```python
from build123d import *

# Parameters (mm, degrees)
SKETCH1_W           = 46
SKETCH1_H           = 21
BOSS_EXTRUDE1_DEPTH = 1
SKETCH2_W           = 21
SKETCH2_H           = 12
SKETCH2_W_2         = 11
SKETCH2_H_2         = 6
BOSS_EXTRUDE2_DEPTH = 4.5
SKETCH3_W           = 7.849871035
SKETCH3_H           = 3.412332869
CUT_EXTRUDE1_DEPTH  = 4
SKETCH4_R           = 5.109251927
BOSS_EXTRUDE3_DEPTH = 3
SKETCH5_R           = 1.986847175
CUT_EXTRUDE2_DEPTH  = 1.5
FILLET1_R           = 1
SKETCH6_R           = 1.1
CUT_EXTRUDE3_DEPTH  = 1.5


with BuildPart() as part:
    # Sketch1 → Boss-Extrude1 (new body)
    with BuildSketch(Plane(origin=(0, 0, 0), x_dir=(1, 0, 0), z_dir=(0, 1, 0))):
        with Locations((23, -10.5)):
            Rectangle(SKETCH1_W, SKETCH1_H)
    extrude(amount=BOSS_EXTRUDE1_DEPTH)

    # Sketch2 → Boss-Extrude2 (add)
    with BuildSketch(Plane(origin=(0, 1, 0), x_dir=(1, 0, 0), z_dir=(0, 1, 0))):
        with Locations((23, -10.5)):
            Rectangle(SKETCH2_W, SKETCH2_H)
        with Locations((39.939580859, -17.520481264)):
            Rectangle(SKETCH2_W_2, SKETCH2_H_2)
    extrude(amount=BOSS_EXTRUDE2_DEPTH)

    # Sketch3 → Cut-Extrude1 (cut)
    with BuildSketch(Plane.XY.offset(20.520481264)):
        with Locations((40.122531197, 3.793833565)):
            Rectangle(SKETCH3_W, SKETCH3_H)
    extrude(amount=-CUT_EXTRUDE1_DEPTH, mode=Mode.SUBTRACT)

    # Sketch4 → Boss-Extrude3 (add)
    with BuildSketch(Plane(origin=(0, 5.5, 0), x_dir=(1, 0, 0), z_dir=(0, 1, 0))):
        with Locations((23.147185082, -10.671715929)):
            Circle(SKETCH4_R)
    extrude(amount=BOSS_EXTRUDE3_DEPTH)

    # Sketch5 → Cut-Extrude2 (cut)
    with BuildSketch(Plane(origin=(0, 8.5, 0), x_dir=(1, 0, 0), z_dir=(0, 1, 0))):
        with Locations((23.147185082, -10.671715929)):
            Circle(SKETCH5_R)
    extrude(amount=-CUT_EXTRUDE2_DEPTH, mode=Mode.SUBTRACT)

    # Fillet1
    fillet1_edges = [part.edges().sort_by_distance(p)[0] for p in [
        (21.160337907, 8.5, 10.671715929),
    ]]
    fillet(fillet1_edges, radius=FILLET1_R)

    # Sketch6 → Cut-Extrude3 (cut)
    with BuildSketch(Plane(origin=(0, 1, 0), x_dir=(1, 0, 0), z_dir=(0, 1, 0))):
        with Locations((1.658163122, -10.5)):
            Circle(SKETCH6_R)
        with Locations((44.341836878, -10.5)):
            Circle(SKETCH6_R)
    extrude(amount=-CUT_EXTRUDE3_DEPTH, mode=Mode.SUBTRACT)


solid = part.part
```
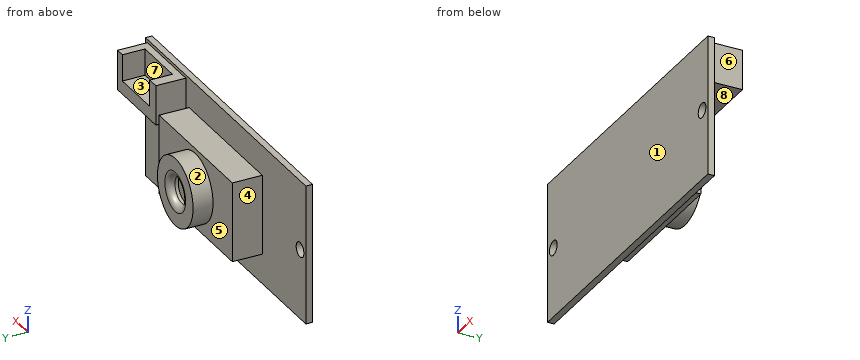
Model file for the job. Use its own axes, mm. Face numbers are marked on the shaded views. A direction names the side the tool comes from. Give positions to 0.01 mm unless a question says otherwise; leave off trailing zeros. Write each loop counter-clockwise with the first axis right and the second up, starting at its lowest first coordinate (ties: lowest second). Pieces come first, ordered by that corner, then holes. Notation, with made-up numbers: M -12,41.5 L 31,41.5 A21 cw 31,71.5 Z; hole C 16,58 d4. An arc over 180 degrees is marked long. Use a Markdown table: item, result.
1) Pin check, flat tips, straight feed: pin 1 (3.5 mm diameter, centred on x = 26.5, y = 4, fed in from +Z); pin 2 (1 mm diameter, centred on y = 6.5, z = 12.5, fed in from -X); pin 3 (2 mm diameter, centred on y = 3.5, z = 17, fed in from -X). Stop position of each tip, or through.
Responses:
| item | result |
|---|---|
| pin 1 | stops at z = 16.5 |
| pin 2 | stops at x = 18.21 |
| pin 3 | stops at x = 12.5 |
2) Cut at C-C (x = 16.5). List the corners of the cut face in (y, z).
Responses:
| item | result |
|---|---|
| outline | M 0,0 L 1,0 L 1,4.5 L 5.5,4.5 L 5.5,16.5 L 1,16.5 L 1,21 L 0,21 Z |
3) Drill centre lines: line 1 (X direction, y = 0.7, z = 10.5); line 2 (X direction, y = 5.25, z = 15.25); line 3 (X direction, y = 3.5, z = 20). Where is each one in solid material? Low to high. Write a range as from..to.
Responses:
| item | result |
|---|---|
| line 1 | x = 0..0.56, 2.76..43.24, 45.44..46 |
| line 2 | x = 12.5..33.5, 34.44..45.44 |
| line 3 | x = 34.44..36.2, 44.05..45.44 |
4) Cut at B-B (z = 5). List the corners of the cut face in (x, y), and give its area (4 significant figures).
Responses:
| item | result |
|---|---|
| outline | M 0,0 L 46,0 L 46,1 L 33.5,1 L 33.5,5.5 L 12.5,5.5 L 12.5,1 L 0,1 Z |
| area | 140.5 mm2 |
5) Cut at D-D (y = 6). List the corners of the cut face in (x, z), and give its area (3 significant figures).
Responses:
| item | result |
|---|---|
| outline | C 23.15,10.67 d10.22 |
| area | 82.0 mm2 |
6) Tool access for the marked faces 4, 5, 6, 7 and 8: list every direction of +Z, -Z, +X, -X, +Y, -Y with a clear straight run to the whole face (end or side of a thin tool).
Responses:
| item | result |
|---|---|
| face 4 | +Z, -Z, -X, +Y |
| face 5 | +Y |
| face 6 | +Z, -Z, +X, +Y |
| face 7 | +Z, +Y |
| face 8 | -Z, +X, +Y |
7) Pull direction X, two halves, no side cores. Call the marked faces 1, 2 and 3: +X half, -X half, draft (parallel to the pull), parting line (faces both ways), or undercut.
Responses:
| item | result |
|---|---|
| face 1 | draft |
| face 2 | parting line |
| face 3 | undercut |
8) Cut at A-A (y = 3.25). List the corners of the cut face in (x, z).
Responses:
| item | result |
|---|---|
| outline | M 12.5,4.5 L 33.5,4.5 L 33.5,16.5 L 12.5,16.5 Z; M 34.44,14.52 L 45.44,14.52 L 45.44,20.52 L 44.05,20.52 L 44.05,16.52 L 36.2,16.52 L 36.2,20.52 L 34.44,20.52 Z |
